from build123d import *

# Parameters (mm, degrees)
F0_W     = 381
F0_H     = 69.85
F0_W_2   = 9.525
F0_H_2   = 12.7
F0_R     = 9.525
F1_DEPTH = 12.7
F2_W     = 50.8
F2_H     = 38.1
F3_DEPTH = 25.4
F4_W     = 50.8
F4_H     = 19.05
F6_R     = 6.35
F7_DEPTH = 76.2


with BuildPart() as f1:
    # F0 (on Top) → F1 (new body)
    with BuildSketch(Plane.XY):
        Rectangle(F0_W, F0_H)
        with Locations((-160.3375, -15.875)):
            Rectangle(F0_W_2, F0_H_2, mode=Mode.SUBTRACT)
        with Locations((160.3375, -15.875)):
            Rectangle(F0_W_2, F0_H_2, mode=Mode.SUBTRACT)
        with Locations((-114.3, 0)):
            Circle(F0_R, mode=Mode.SUBTRACT)
        with Locations((-71.4375, 15.875)):
            Rectangle(F0_W_2, F0_H_2, mode=Mode.SUBTRACT)
        with Locations((71.4375, 15.875)):
            Rectangle(F0_W_2, F0_H_2, mode=Mode.SUBTRACT)
        with Locations((114.3, 0)):
            Circle(F0_R, mode=Mode.SUBTRACT)
    extrude(amount=F1_DEPTH)

    # F2 (on face) → F3 (join)
    with BuildSketch(Plane(origin=(0, 0, 0), x_dir=(1, 0, 0), z_dir=(0, 0, -1))):
        Rectangle(F2_W, F2_H)
    extrude(amount=F3_DEPTH)

    # F4 (on face) → F5 (revolve)
    with BuildSketch(Plane(origin=(0, 0, -25.4), x_dir=(1, 0, 0), z_dir=(0, 0, -1))):
        with Locations((0, -9.525)):
            Rectangle(F4_W, F4_H)
    revolve(axis=Axis((0, 0, -25.4), (1, 0, 0)))

    # F6 (on face) → F7 (cut)
    with BuildSketch(Plane(origin=(-25.4, 0, 0), x_dir=(0, -1, 0), z_dir=(-1, 0, 0))):
        with Locations((0, -25.4)):
            Circle(F6_R)
    extrude(amount=-F7_DEPTH, mode=Mode.SUBTRACT)


solid = f1.part
Part model, mm, in its own coordinate system. A direction names the side the tool comes from. Round coordinates to 2 decimals unless told otherwise and drop trailing zeros. Loops run counter-clockwise (first coordinate to the right, second up) from the corner with the lowest first, then second, coordinate; pieces in that order, holes last. Notation, with made-up numbers: (22, -39.75) - (70, -39.75) arc R21 ccw to (70, -22.75) - close; hole circle Ø3 at (-40, -7.5). An arc over 180 degrees is marked (long way). Answer as a JSON object with one key per item and string values.
Item 1: Band-saw the part on D-D on y = -30. List the corners of the cut face in (x, z), plus the area to 3 significant figures.
Output:
{"outline": "(-190.5, 0) - (190.5, 0) - (190.5, 12.7) - (-190.5, 12.7) - close", "area": "4,840 mm2"}
Item 2: Band-saw the part on A-A on x = -114.3. List the corners of the cut face in (y, z) (3 decimals).
Output:
{"outline": "(-34.925, 0) - (-9.525, 0) - (-9.525, 12.7) - (-34.925, 12.7) - close; (9.525, 0) - (34.925, 0) - (34.925, 12.7) - (9.525, 12.7) - close"}
Item 3: Pull direction X, two halves, no side cores. Call faces 1 (the face through (-66.675, 16, 6)), 2 (the face through (25.4, 0, -17)), 3 (the face through (0.356, -0.419, -44.445)), 4 (the face through (-160, -9.525, 6)): pulls with the +X half, pulls with the -X half, needs draft (parallel to the pull), parting line crosses it, or undercut.
Output:
{"face 1": "undercut", "face 2": "pulls with the +X half", "face 3": "needs draft", "face 4": "undercut"}
Item 4: Wall check: L1, parallel to Y at x = -114, z = 8 (3 decimals); L2, parallel to Z at x = -61.5, y = 31.5; L3, parallel to X at y = 5.5, z = -30. Give the ranges that are in metal, low to high.
Output:
{"L1": "-34.925 to -9.52, 9.52 to 34.925", "L2": "0 to 12.7", "L3": "-25.4 to 25.4"}
Item 5: Band-saw the part on C-C on z = -10.5. List the corners of the cut face in (x, y).
Output:
{"outline": "(-25.4, -19.05) - (25.4, -19.05) - (25.4, 19.05) - (-25.4, 19.05) - close"}
Item 6: Pin check, flat tips, straight feed: pin 1 (8 mm diameter, centred on y = 16.5, z = -7.5, fed in from +X); pin 2 (4 mm diameter, centred on y = -10.5, z = -24.5, fed in from -X); pin 3 (1.5 mm diameter, centred on x = 107, y = -8.5, fed in from -Z). Stop position of each tip, or through.
Output:
{"pin 1": "x = 25.4", "pin 2": "x = -25.4", "pin 3": "z = 0"}
Item 7: Band-saw the part on B-B on y = 0. List the corners of the cut face in (x, z) (3 decimals), plus the area to 3 significant figures.
Output:
{"outline": "(-190.5, 0) - (-123.825, 0) - (-123.825, 12.7) - (-190.5, 12.7) - close; (-104.775, 0) - (-25.4, 0) - (-25.4, -19.05) - (25.4, -19.05) - (25.4, 0) - (104.775, 0) - (104.775, 12.7) - (-104.775, 12.7) - close; (-25.4, -44.45) - (25.4, -44.45) - (25.4, -31.75) - (-25.4, -31.75) - close; (123.825, 0) - (190.5, 0) - (190.5, 12.7) - (123.825, 12.7) - close", "area": "5,970 mm2"}
Item 8: Tool access for faces 5 (the face through (-25.4, 0, -17)), 6 (the face through (0, -19.05, -13)), 7 (the face through (-190.5, 0, 6)), 8 (the face through (165.1, -16, 6)), 9 (the face through (-3, 0, 12.7)): list every direction of +Z, -Z, +X, -X, +Y, -Y with a clear straight run to the whole face (end or side of a thin tool).
Output:
{"face 5": "-Z, -X, +Y, -Y", "face 6": "-Z, +X, -X, -Y", "face 7": "+Z, -Z, -X, +Y, -Y", "face 8": "+Z, -Z", "face 9": "+Z, +X, -X, +Y, -Y"}
